Input: dimensioned drawing with shaded views. Units: mm. Origin: part minimum x, y, z. Coordinates: 2 decimals unless noted, no trailing zeros. Order: outer loops, then holes, each group sorted by start corner. A loop starts at its lowest first (then second) coordinate and runs counter-clockwise, first axis right, second up.
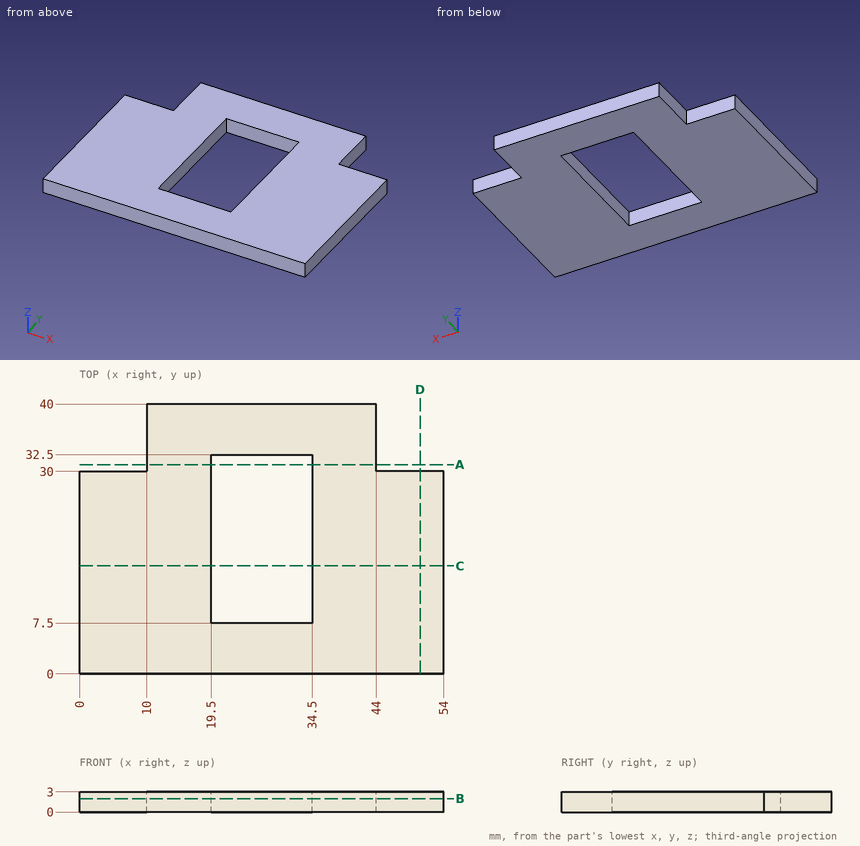
1. Section query A-A, the plane y = 31. Output: boundary loops of the cut face in (x, z), plus the area to 3 significant figures.
2. Section query C-C, the plane y = 16. Output: boundary loops of the cut face in (x, z).
3. Section query D-D, the plane x = 50.5. Output: boundary loops of the cut face in (y, z).
4. Section query B-B, the plane z = 2. Output: boundary loops of the cut face in (x, y), plus the area to 4 significant figures.
5. Contact query for flat-ended pins moving along their axis: P1, Ø1.5, axis at y = 20.5, z = 2, coming from the -X side; P2, Ø1.5, axis at x = 4.5, z = 1, coming from the +Y side; P3, Ø0.9, axis at y = 33, z = 1.5, coming from the -X side. Output: stop coordinate, or through.
6. Material intervals for line 1 along X through (y, z) = (15, 2.2); line 2 along X through (y, z) = (31.5, 0.8); line 3 along Y through (x, z) = (27, 1.4), sorted ascending.
Answer key:
1. outline: (10, 0) - (19.5, 0) - (19.5, 3) - (10, 3) - close; (34.5, 0) - (44, 0) - (44, 3) - (34.5, 3) - close
1. area: 57.0 mm2
2. outline: (0, 0) - (19.5, 0) - (19.5, 3) - (0, 3) - close; (34.5, 0) - (54, 0) - (54, 3) - (34.5, 3) - close
3. outline: (0, 0) - (30, 0) - (30, 3) - (0, 3) - close
4. outline: (0, 0) - (54, 0) - (54, 30) - (44, 30) - (44, 40) - (10, 40) - (10, 30) - (0, 30) - close; hole (19.5, 7.5) - (34.5, 7.5) - (34.5, 32.5) - (19.5, 32.5) - close
4. area: 1,585 mm2
5. P1: stops at x = 0
5. P2: stops at y = 30
5. P3: stops at x = 10
6. line 1: x = 0 to 19.5, 34.5 to 54
6. line 2: x = 10 to 19.5, 34.5 to 44
6. line 3: y = 0 to 7.5, 32.5 to 40
